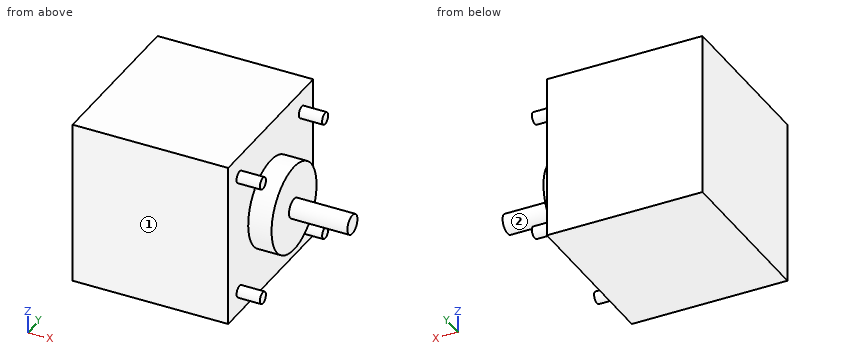
```python
from build123d import *

# Parameters (mm, degrees)
CYLINDER231_R     = 1.5
CYLINDER231_DEPTH = 6
CYLINDER229_R     = 1.5
CYLINDER229_DEPTH = 6
CYLINDER227_R     = 11.2
CYLINDER227_DEPTH = 6
CYLINDER_R        = 2.5
CYLINDER_DEPTH    = 21
CYLINDER230_R     = 1.5
CYLINDER230_DEPTH = 6
CYLINDER228_R     = 1.5
CYLINDER228_DEPTH = 6
BOX_W             = 40
BOX_H             = 42.3
BOX_DEPTH         = 42.3


with BuildPart() as cylinder231:
    # Cylinder231 → Cylinder231 (new body)
    with BuildSketch(Plane(origin=(40, 5.65, 36.665), x_dir=(0, 0, -1), z_dir=(1, 0, 0))):
        Circle(CYLINDER231_R)
    extrude(amount=CYLINDER231_DEPTH)


with BuildPart() as cylinder229:
    # Cylinder229 → Cylinder229 (new body)
    with BuildSketch(Plane(origin=(40, 36.65, 36.65), x_dir=(0, 0, -1), z_dir=(1, 0, 0))):
        Circle(CYLINDER229_R)
    extrude(amount=CYLINDER229_DEPTH)


with BuildPart() as cylinder227:
    # Cylinder227 → Cylinder227 (new body)
    with BuildSketch(Plane(origin=(40, 21.15, 21.15), x_dir=(0, 0, -1), z_dir=(1, 0, 0))):
        Circle(CYLINDER227_R)
    extrude(amount=CYLINDER227_DEPTH)


with BuildPart() as cylinder:
    # Cylinder → Cylinder (new body)
    with BuildSketch(Plane(origin=(40, 21.15, 21.15), x_dir=(0, 0, -1), z_dir=(1, 0, 0))):
        Circle(CYLINDER_R)
    extrude(amount=CYLINDER_DEPTH)


with BuildPart() as cylinder230:
    # Cylinder230 → Cylinder230 (new body)
    with BuildSketch(Plane(origin=(40, 5.65, 5.65), x_dir=(0, 0, -1), z_dir=(1, 0, 0))):
        Circle(CYLINDER230_R)
    extrude(amount=CYLINDER230_DEPTH)


with BuildPart() as cylinder228:
    # Cylinder228 → Cylinder228 (new body)
    with BuildSketch(Plane(origin=(40, 36.65, 5.65), x_dir=(0, 0, -1), z_dir=(1, 0, 0))):
        Circle(CYLINDER228_R)
    extrude(amount=CYLINDER228_DEPTH)


with BuildPart() as fusion:
    # Box → Box (new body)
    with BuildSketch(Plane.XY):
        with Locations((20, 21.15)):
            Rectangle(BOX_W, BOX_H)
    extrude(amount=BOX_DEPTH)

    # Fusion: union Cylinder231, Cylinder229, Cylinder227, Cylinder, Cylinder230, Cylinder228
    add(cylinder231.part)
    add(cylinder229.part)
    add(cylinder227.part)
    add(cylinder.part)
    add(cylinder230.part)
    add(cylinder228.part)


with BuildPart() as fusion_1:
    # Fusion placement: moved
    add(fusion.part.moved(Location((59.2, -37.4, 49.3))))


solid = fusion_1.part
```
The listing builds one solid part. Answer for the finished solid, in the listing's coordinates (mm). Face numbers are marked on the shaded views. A direction names the side the tool comes from. Coordinates: 2 decimals unless noted, no trailing zeros. Order: outer loops, then holes, each group sorted by start corner. A loop starts at its lowest first (then second) coordinate and runs counter-clockwise, first axis right, second up. Notation, with made-up numbers: M -23,-3.5 L 0,-3.5 A25 cw 0,33.5 Z; hole C 35,-14 d3. An arc over 180 degrees is marked long. Answer as a JSON object with one key per item and string values. Group by question number.
1. Section D-D on y = -26 is taken. Write down the section's boundary in (x, z).
2. Straight lines are drawn through the part: line 1 (Y direction, x = 104.5, z = 55); line 2 (X direction, y = -34.5, z = 68.5); line 3 (X direction, y = -14.5, z = 67.5). For each, find the intervals that lie inside material, in ascending order.
3. Section B-B on z = 70.45 is taken. Write down the section's boundary in (x, y), then the cut area to 3 significant figures.
4. Flat-ended cylindrical pins translate along their axes: P1, Ø0.9, axis at y = -32, z = 86.5, coming from the +X side; P2, Ø3, axis at y = -22, z = 57, coming from the +X side; P3, Ø1, axis at x = 100, y = -8, coming from the -Z side. Find the tip coordinate at first contact, or state that the pin passes through.
5. Section A-A on x = 100 is taken. Write down the section's boundary in (y, z) (3 decimals).
6. A tool of negligible diameter and unlimited length cuts with its end or side. For the marked faces 1 and 2, from which of +Z, -Z, +X, -X, +Y, -Y can it reach the whole face along a straight path? Write none if from no direction.
7. Section C-C on y = -16.25 is taken. Write down the section's boundary in (x, z), then the cut area to 3 significant figures.
Values follow:
{
 "1": {"outline": "M 59.2,49.3 L 99.2,49.3 L 99.2,64.94 L 105.2,64.94 L 105.2,75.96 L 99.2,75.96 L 99.2,91.6 L 59.2,91.6 Z"},
 "2": {"line 1": "-33.25 to -30.25, -2.25 to 0.75", "line 2": "59.2 to 99.2", "line 3": "59.2 to 105.2"},
 "3": {"outline": "M 59.2,-37.4 L 99.2,-37.4 L 99.2,-27.45 L 105.2,-27.45 L 105.2,-18.75 L 120.2,-18.75 L 120.2,-13.75 L 105.2,-13.75 L 105.2,-5.05 L 99.2,-5.05 L 99.2,4.9 L 59.2,4.9 Z", "area": "1,900 mm2"},
 "4": {"P1": "x = 105.2", "P2": "x = 99.2", "P3": "z = 62.36"},
 "5": {"outline": "C -31.75,54.95 d3; C -31.75,85.965 d3; C -16.25,70.45 d22.4; C -0.75,54.95 d3; C -0.75,85.95 d3"},
 "6": {"face 1": "+Z, -Z, +X, -X, -Y", "face 2": "+X"},
 "7": {"outline": "M 59.2,49.3 L 99.2,49.3 L 99.2,59.25 L 105.2,59.25 L 105.2,67.95 L 120.2,67.95 L 120.2,72.95 L 105.2,72.95 L 105.2,81.65 L 99.2,81.65 L 99.2,91.6 L 59.2,91.6 Z", "area": "1,900 mm2"}
}
